from build123d import *


with BuildPart() as part:
    # Sketch1 → Revolve1 (revolve)
    with BuildSketch(Plane.XY, mode=Mode.PRIVATE) as revolve1_sk:
        with BuildLine():
            Line((0, 0), (-59.5, 0))
            ThreePointArc((-59.5, 0), (-61.621320344, 0.878679656), (-62.5, 3))
            Line((-62.5, 3), (-62.5, 129))
            ThreePointArc((-62.5, 129), (-63.378679656, 131.121320344), (-65.5, 132))
            Line((-65.5, 132), (-67.983599332, 132))
            ThreePointArc((-67.983599332, 132), (-69.983599332, 134), (-67.983599332, 136))
            Line((-67.983599332, 136), (-65.5, 136))
            ThreePointArc((-65.5, 136), (-60.550252532, 133.949747468), (-58.5, 129))
            Line((-58.5, 129), (-58.5, 4))
            Line((-58.5, 4), (0, 4))
            Line((0, 4), (0, 0))
        make_face()
    revolve(revolve1_sk.sketch.rotate(Axis((0, 0, 0), (0, 1, 0)), 270), axis=Axis((0, 0, 0), (0, 1, 0)))


solid = part.part
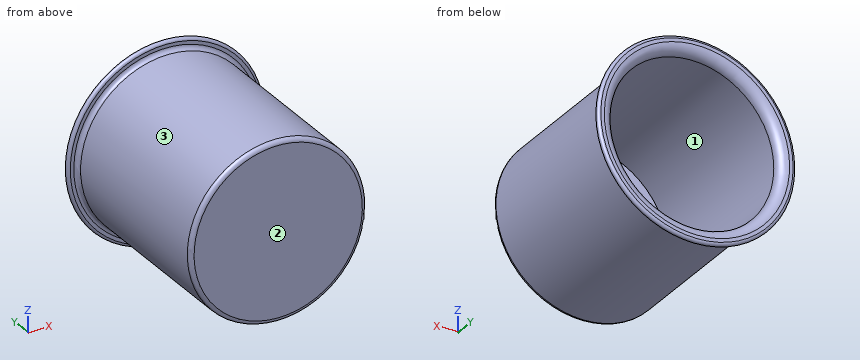
Model file for the job. Use its own axes, mm. Face numbers are marked on the shaded views. Give positions to 0.01 mm unless a question says otherwise; leave off trailing zeros. Write each loop counter-clockwise with the first axis right and the second up, starting at its lowest first coordinate (ties: lowest second). Pieces come first, ordered by that corner, then holes. Notation, with made-up numbers: (-20.5, 6) -> (-8.5, 6) arc R19 ccw to (-8.5, 29) -> close; hole circle Ø11 at (18, 61.5). An arc over 180 degrees is marked (long way). Write item = value, one per line.
(1) Mould opens along Z. For the marked faces 1, 2 and 3 say: released by +Z, released by -Z, zero draft, split by the parting line, or undercut.
Determined:
face_1 = undercut
face_2 = zero draft
face_3 = split by the parting line
(2) Flat gauge pins, fed straight in: P1, Ø5, axis at x = -29, y = 67.5, coming from the +Z side; P2, Ø4, axis at x = -15.5, z = 2, coming from the +Y side; P3, Ø1, axis at y = 61, z = -13.5, coming from the +X side. Where does each tip first touch, or does it go through?
Determined:
P1 = 56.6
P2 = 4
P3 = 61.13
(3) Slice it at C-C, the plane y = 82.5. Give the cut face in (x, z), then the cut area to 3 significant figures.
Determined:
outline = circle Ø125 at (0, 0); hole circle Ø117 at (0, 0)
area = 1,520 mm2
(4) Slice it at A-A, the plane x = 0. Give the cut face in (y, z), then the cut area to 3 significant figures.
Determined:
outline = (0, -59.5) arc R3 ccw to (3, -62.5) -> (129, -62.5) arc R3 cw to (132, -65.5) -> (132, -67.98) arc R2 ccw to (136, -67.98) -> (136, -65.5) arc R7 ccw to (129, -58.5) -> (4, -58.5) -> (4, 58.5) -> (129, 58.5) arc R7 ccw to (136, 65.5) -> (136, 67.98) arc R2 ccw to (132, 67.98) -> (132, 65.5) arc R3 cw to (129, 62.5) -> (3, 62.5) arc R3 ccw to (0, 59.5) -> close
area = 1,590 mm2
(5) Probe line 1 along X through (y, z) = (48, 0); line 2 along X through (y, z) = (27, -19.5); line 3 along Z through (x, y) = (40, 99). List the from-to ranges inside material, lowest first.
Determined:
line_1 = -62.5 to -58.5, 58.5 to 62.5
line_2 = -59.38 to -55.15, 55.15 to 59.38
line_3 = -48.02 to -42.69, 42.69 to 48.02
(6) Slice it at B-B, the plane z = 0. Give the cut face in (x, y).
Determined:
outline = (-67.98, 132) -> (-65.5, 132) arc R3 cw to (-62.5, 129) -> (-62.5, 3) arc R3 ccw to (-59.5, 0) -> (59.5, 0) arc R3 ccw to (62.5, 3) -> (62.5, 129) arc R3 cw to (65.5, 132) -> (67.98, 132) arc R2 ccw to (67.98, 136) -> (65.5, 136) arc R7 ccw to (58.5, 129) -> (58.5, 4) -> (-58.5, 4) -> (-58.5, 129) arc R7 ccw to (-65.5, 136) -> (-67.98, 136) arc R2 ccw to start
